The listing builds one solid part. Answer for the finished solid, in the listing's coordinates (mm). A direction names the side the tool comes from. Round coordinates to 2 decimals unless told otherwise and drop trailing zeros. Order: outer loops, then holes, each group sorted by start corner. A loop starts at its lowest first (then second) coordinate and runs counter-clockwise, first axis right, second up. Notation, with made-up numbers: (-22, 19.5) - (-14, 19.5) arc R25 cw to (-14, 39.5) - close; hole circle Ø4 at (72.25, 50). An arc over 180 degrees is marked (long way). Write item = value, one per line.
from build123d import *

# Parameters (mm, degrees)
SKETCH2_R                       = 48.5
BOSS_EXTRUDE1_DEPTH             = 4
SKETCH4_R                       = 1.5
CUT_EXTRUDE2_DEPTH              = 69.705894944
SKETCH5_R                       = 2.5
CUT_EXTRUDE3_DEPTH              = 69.705894944
BOSS_EXTRUDE2_DEPTH             = 14
CUT_EXTRUDE5_REACH              = 97.597
SKETCH9_R                       = 1.3
CUT_EXTRUDE6_DEPTH              = 7.5
CUT_EXTRUDE9_REACH              = 96.471
SKETCH11_R                      = 9
BOSS_EXTRUDE7_DEPTH             = 9
BOSS_EXTRUDE7_DIRECTION_2_REACH = 104.912
BOSS_EXTRUDE10_DEPTH            = 9
SKETCH27_W                      = 16
SKETCH27_H                      = 6
BOSS_EXTRUDE11_DEPTH            = 12
FILLET6_R                       = 3
CUT_EXTRUDE16_REACH             = 111.016
SKETCH28_W                      = 8
SKETCH28_H                      = 4
CUT_EXTRUDE17_DEPTH             = 95.342420983
CUT_EXTRUDE17_DEPTH_BACK        = 95.342420983


with BuildPart() as part:
    # Sketch2 → Boss-Extrude1 (new body)
    with BuildSketch(Plane(origin=(0, 0, 0), x_dir=(1, 0, 0), z_dir=(0, 1, 0))):
        with Locations(Location((0, 0, 0), (0, 0, 270))):
            Circle(SKETCH2_R)
    extrude(amount=BOSS_EXTRUDE1_DEPTH)

    # Sketch4 → Cut-Extrude2 (cut, through all)
    with BuildSketch(Plane.XZ):
        with Locations(Location((0, 7.25, 0), (0, 0, 270))):
            Circle(SKETCH4_R)
        with Locations(Location((0, -7.25, 0), (0, 0, 270))):
            Circle(SKETCH4_R)
    extrude(amount=-CUT_EXTRUDE2_DEPTH, mode=Mode.SUBTRACT)

    # Sketch5 → Cut-Extrude3 (cut, through all)
    with BuildSketch(Plane.XZ):
        with Locations(Location((0, 0, 0), (0, 0, 270))):
            Circle(SKETCH5_R)
    extrude(amount=-CUT_EXTRUDE3_DEPTH, mode=Mode.SUBTRACT)

    # Sketch7 → Boss-Extrude2 (add)
    with BuildSketch(Plane(origin=(-4, 0, 0), x_dir=(0, 0, -1), z_dir=(1, 0, 0))):
        with BuildLine():
            Line((23.129947874, 4), (23.129947874, 11.644549616))
            ThreePointArc((23.129947874, 11.644549616), (24.589048403, 18.743749901), (28.729797284, 24.692011643))
            ThreePointArc((28.729797284, 24.692011643), (29.313383054, 55.284736897), (-1.284289494, 55.479275971))
            Line((-1.284289494, 55.479275971), (-27.227315747, 29.536249718))
            ThreePointArc((-27.227315747, 29.536249718), (-32.64663453, 21.425665997), (-34.549646217, 11.858580188))
            Line((-34.549646217, 11.858580188), (-34.549646217, 4))
            Line((-34.549646217, 4), (23.129947874, 4))
        make_face()
    extrude(amount=-BOSS_EXTRUDE2_DEPTH)

    # Sketch8 → Cut-Extrude5 (cut, up to next)
    with BuildSketch(Plane(origin=(-6, 0, 0), x_dir=(0, 0, -1), z_dir=(1, 0, 0)), mode=Mode.PRIVATE) as cut_extrude5_sk1:
        Polygon((-15.249648422, 25.957567857), (13.741729607, 54.948945886), (28.590972012, 40.099703481), (-0.400406017, 11.108325452), align=None)
    cut_extrude5_tool1 = extrude(cut_extrude5_sk1.sketch, amount=-CUT_EXTRUDE5_REACH, mode=Mode.PRIVATE) & part.part
    add(cut_extrude5_tool1.solids().sort_by_distance((-6, 33.028636, -6.670662))[0], mode=Mode.SUBTRACT)

    # Sketch9 → Cut-Extrude6 (cut)
    with BuildSketch(Plane.ZY.offset(18)):
        with Locations((-20.105690637, 53.534732323)):
            Circle(SKETCH9_R)
        with Locations((-27.176758449, 46.463664511)):
            Circle(SKETCH9_R)
        with Locations((6.764367048, 12.522539014)):
            Circle(SKETCH9_R)
        with Locations((13.83543486, 19.593606826)):
            Circle(SKETCH9_R)
    extrude(amount=-CUT_EXTRUDE6_DEPTH, mode=Mode.SUBTRACT)

    # Sketch11 → Cut-Extrude9 (cut, up to next)
    with BuildSketch(Plane(origin=(-4, 0, 0), x_dir=(0, 0, -1), z_dir=(1, 0, 0)), mode=Mode.PRIVATE) as cut_extrude9_sk1:
        with Locations((13.918506302, 40.276480176)):
            Circle(SKETCH11_R)
    cut_extrude9_tool1 = extrude(cut_extrude9_sk1.sketch, amount=-CUT_EXTRUDE9_REACH, mode=Mode.PRIVATE) & part.part
    add(cut_extrude9_tool1.solids().sort_by_distance((-4, 40.27648, -13.918506))[0], mode=Mode.SUBTRACT)

    # Sketch17 → Boss-Extrude7 (add)
    with BuildSketch(Plane.ZY.offset(18)):
        with BuildLine():
            ThreePointArc((34.549646217, 11.858580188), (33.008342843, 20.500891953), (28.574482006, 28.077569775))
            ThreePointArc((28.574482006, 28.077569775), (27.915386359, 28.820289685), (27.227315747, 29.536249718))
            Line((27.227315747, 29.536249718), (1.284289494, 55.479275971))
            Line((1.284289494, 55.479275971), (26.295003593, 26.127182305))
            ThreePointArc((26.295003593, 26.127182305), (30.194232218, 19.461281607), (31.549646217, 11.858580188))
            Line((31.549646217, 11.858580188), (31.549646217, 4))
            Line((31.549646217, 4), (34.549646217, 4))
            Line((34.549646217, 4), (34.549646217, 11.858580188))
        make_face()
        with BuildLine():
            Line((28.574482006, 28.077569775), (3.405609837, 57.600596315))
            ThreePointArc((3.405609837, 57.600596315), (-31.461505391, 57.378912253), (-30.796489049, 22.517434639))
            ThreePointArc((-30.796489049, 22.517434639), (-27.345864981, 17.560549854), (-26.129947874, 11.644549616))
            Line((-26.129947874, 11.644549616), (-26.129947874, 4))
            Line((-26.129947874, 4), (-23.129947874, 4))
            Line((-23.129947874, 4), (-23.129947874, 11.644549616))
            ThreePointArc((-23.129947874, 11.644549616), (-24.589048403, 18.743749901), (-28.729797284, 24.692011643))
            ThreePointArc((-28.729797284, 24.692011643), (-29.313383054, 55.284736897), (1.284289494, 55.479275971))
            Line((1.284289494, 55.479275971), (27.227315747, 29.536249718))
            ThreePointArc((27.227315747, 29.536249718), (27.915386359, 28.820289685), (28.574482006, 28.077569775))
        make_face()
    extrude(amount=BOSS_EXTRUDE7_DEPTH)

    # Boss-Extrude7 direction 2: up to this face of the body (flat: up to its plane)
    boss_extrude7_direction_2_end = Plane(part.part.faces().sort_by_distance((-4, 28.276431801, -1.649713195))[0])
    # Sketch17 → Boss-Extrude7 direction 2 (add, up to the picked face)
    with BuildSketch(Plane.ZY.offset(18), mode=Mode.PRIVATE) as boss_extrude7_direction_2_sk1:
        with BuildLine():
            ThreePointArc((34.549646217, 11.858580188), (33.008342843, 20.500891953), (28.574482006, 28.077569775))
            ThreePointArc((28.574482006, 28.077569775), (27.915386359, 28.820289685), (27.227315747, 29.536249718))
            Line((27.227315747, 29.536249718), (1.284289494, 55.479275971))
            Line((1.284289494, 55.479275971), (26.295003593, 26.127182305))
            ThreePointArc((26.295003593, 26.127182305), (30.194232218, 19.461281607), (31.549646217, 11.858580188))
            Line((31.549646217, 11.858580188), (31.549646217, 4))
            Line((31.549646217, 4), (34.549646217, 4))
            Line((34.549646217, 4), (34.549646217, 11.858580188))
        make_face()
    boss_extrude7_direction_2_tool1 = split(extrude(boss_extrude7_direction_2_sk1.sketch, amount=-BOSS_EXTRUDE7_DIRECTION_2_REACH, mode=Mode.PRIVATE), bisect_by=boss_extrude7_direction_2_end, keep=Keep.BOTH, mode=Mode.PRIVATE)
    # Sketch17 → Boss-Extrude7 direction 2 (add, up to the picked face)
    with BuildSketch(Plane.ZY.offset(18), mode=Mode.PRIVATE) as boss_extrude7_direction_2_sk2:
        with BuildLine():
            Line((28.574482006, 28.077569775), (3.405609837, 57.600596315))
            ThreePointArc((3.405609837, 57.600596315), (-31.461505391, 57.378912253), (-30.796489049, 22.517434639))
            ThreePointArc((-30.796489049, 22.517434639), (-27.345864981, 17.560549854), (-26.129947874, 11.644549616))
            Line((-26.129947874, 11.644549616), (-26.129947874, 4))
            Line((-26.129947874, 4), (-23.129947874, 4))
            Line((-23.129947874, 4), (-23.129947874, 11.644549616))
            ThreePointArc((-23.129947874, 11.644549616), (-24.589048403, 18.743749901), (-28.729797284, 24.692011643))
            ThreePointArc((-28.729797284, 24.692011643), (-29.313383054, 55.284736897), (1.284289494, 55.479275971))
            Line((1.284289494, 55.479275971), (27.227315747, 29.536249718))
            ThreePointArc((27.227315747, 29.536249718), (27.915386359, 28.820289685), (28.574482006, 28.077569775))
        make_face()
    boss_extrude7_direction_2_tool2 = split(extrude(boss_extrude7_direction_2_sk2.sketch, amount=-BOSS_EXTRUDE7_DIRECTION_2_REACH, mode=Mode.PRIVATE), bisect_by=boss_extrude7_direction_2_end, keep=Keep.BOTH, mode=Mode.PRIVATE)
    add(boss_extrude7_direction_2_tool1.solids().sort_by(Axis((-18, 4.612919, 33.049646), (1, 0, 0)))[0])
    add(boss_extrude7_direction_2_tool2.solids().sort_by(Axis((-18, 43.147366, 14.895406), (1, 0, 0)))[0])

    # Sketch25 → Boss-Extrude10 (add)
    with BuildSketch(Plane.ZY.offset(18)):
        with BuildLine():
            ThreePointArc((-28.729797284, 24.692011643), (-24.589048403, 18.743749901), (-23.129947874, 11.644549616))
            Line((-23.129947874, 11.644549616), (-23.129947874, 4))
            Line((-23.129947874, 4), (-15.129947874, 4))
            add(Edge.make_bspline(
                [(-28.729797284, 24.692011643), (-21.954867515, 18.253200081), (-19.09405247, 12.798017691), (-15.129947874, 4)],
                knots=[0, 0, 0, 0, 1, 1, 1, 1], degree=3))
        make_face()
        with BuildLine():
            add(Edge.make_bspline(
                [(11.751619577, 43.19501844), (26.551255916, 25.8264495), (25.549646217, 4)],
                knots=[0, 0, 0, 1, 1, 1], degree=2))
            Line((25.549646217, 4), (31.549646217, 4))
            Line((31.549646217, 4), (31.549646217, 11.858580188))
            ThreePointArc((31.549646217, 11.858580188), (30.194232218, 19.461281607), (26.295003593, 26.127182305))
            Line((26.295003593, 26.127182305), (11.751619577, 43.19501844))
        make_face()
    extrude(amount=BOSS_EXTRUDE10_DEPTH)

    # Sketch27 → Boss-Extrude11 (add)
    with BuildSketch(Plane(origin=(0, 4, 0), x_dir=(1, 0, 0), z_dir=(0, 1, 0))):
        with Locations((6, -21.549646217)):
            Rectangle(SKETCH27_W, SKETCH27_H)
    extrude(amount=BOSS_EXTRUDE11_DEPTH)

    # Fillet6
    fillet6_edges = [part.edges().sort_by_distance(p)[0] for p in [
        (-2, 16, 21.549646217),
        (14, 16, 21.549646217),
    ]]
    fillet(fillet6_edges, radius=FILLET6_R)

    # Sketch28 → Cut-Extrude16 (cut, up to next)
    with BuildSketch(Plane.XY.offset(24.549646217), mode=Mode.PRIVATE) as cut_extrude16_sk1:
        with Locations((6, 10)):
            Rectangle(SKETCH28_W, SKETCH28_H)
    cut_extrude16_tool1 = extrude(cut_extrude16_sk1.sketch, amount=-CUT_EXTRUDE16_REACH, mode=Mode.PRIVATE) & part.part
    add(cut_extrude16_tool1.solids().sort_by_distance((6, 10, 24.549646))[0], mode=Mode.SUBTRACT)

    # Sketch29 → Cut-Extrude17 (cut, two sides: drawn at the far end of the back side and taken through both)
    with BuildSketch(Plane.XY.offset(-CUT_EXTRUDE17_DEPTH_BACK)):
        with BuildLine():
            Line((-21, 64.776480176), (-27, 64.776480176))
            Line((-27, 64.776480176), (-27, 4))
            Line((-27, 4), (-26.5, 4))
            add(Edge.make_bspline(
                [(-21, 64.776480176), (-21.220459696, 34.140901434), (-26.5, 4)],
                knots=[0, 0, 0, 1, 1, 1], degree=2))
        make_face()
    extrude(amount=CUT_EXTRUDE17_DEPTH + CUT_EXTRUDE17_DEPTH_BACK, mode=Mode.SUBTRACT)


solid = part.part
Q1. Section D-D on x = -32 is taken. Determine the outline of the cut face in (y, z), then the cut area to 3 significant figures.
Model answer:
outline = (0, -36.45) - (4, -36.45) - (4, 36.45) - (0, 36.45) - close
area = 292 mm^2
Q2. Flat-ended cylindrical pins translate along their axes: P1, Ø6.5, axis at x = 4.5, z = 22.5, coming from the +Y side; P2, Ø3, axis at y = 10, z = 21.5, coming from the -X side; P3, Ø23.5, axis at y = 40.28, z = -13.92, coming from the +X side; P4, Ø3, axis at x = 19.5, z = -2, coming from the -Y side. Find the tip coordinate at first contact, or state that the pin passes through.
Model answer:
P1 = 16
P2 = -18
P3 = -4
P4 = 0
Q3. Determine the mould class of faces 5 (the face through (6, 8, 22)), 6 (the face through (-10, 0, -1)), 7 (the face through (-11.92, 18.43, 7.72)), 8 (the face through (-15, 8, 34.55)) for opening direction Y: released by +Y, released by -Y, zero draft, split by the parting line, or undercut.
Model answer:
face_5 = undercut
face_6 = released by -Y
face_7 = undercut
face_8 = zero draft
Q4. Section B-B on z = -7.25 is taken. Count the separate pieces of the cut face and the enclosed holes in it, then the cut area to 3 significant figures.
Model answer:
separate_pieces = 3
enclosed_holes = 0
area = 838 mm^2
Q5. Section C-C on x = 23 is taken. Determine the outline of the cut face in (y, z), then the cut area to 3 significant figures.
Model answer:
outline = (0, -42.7) - (4, -42.7) - (4, 42.7) - (0, 42.7) - close
area = 342 mm^2
Q6. For faces 1 (the face through (-10.5, 54, -20)), 2 (the face through (-2.44, 1.97, 0.54)), 3 (the face through (10, 10, 22)), 4 (the face through (-14.77, 17.64, -27.38)), determine the directions among +Z, -Z, +X, -X, +Y, -Y from which every point of the face is accessible in a straight line to the end or side of a thin tool.
Model answer:
face_1 = -X
face_2 = +Y, -Y
face_3 = +Z, -Z
face_4 = -Z, +X, -X
Q7. Section A-A on x = -12 is taken. Determine the outline of the cut face in (y, z), then the cut area to 3 significant figures.
Model answer:
outline = (0, -46.99) - (4, -46.99) - (4, -26.13) - (11.64, -26.13) arc R15 cw to (22.52, -30.8) arc R24.5 ccw (long way) to (57.6, 3.41) - (28.08, 28.57) arc R25 ccw to (11.86, 34.55) - (4, 34.55) - (4, 46.99) - (0, 46.99) - close; hole (11.11, 0.4) - (40.1, -28.59) - (54.95, -13.74) - (25.96, 15.25) - close; hole circle Ø2.6 at (12.52, 6.76); hole circle Ø2.6 at (19.59, 13.84); hole circle Ø2.6 at (46.46, -27.18); hole circle Ø2.6 at (53.53, -20.11)
area = 2,710 mm^2
Q8. Find the intervals of material crossed by line 1 (Y direction, x = 4, z = -42.5); line 2 (Y direction, x = -20.5, z = -31); line 3 (X direction, y = 51, z = -32.5), in increasing order. Write a range as from..to.
Model answer:
line_1 = 0..4
line_2 = 0..4, 22.71..27.22, 53.33..57.84
line_3 = -18..-4
